from build123d import *

# Parameters (mm, degrees)
F1_DEPTH  = 38
F3_D      = 12
F5_DEPTH  = 2
F6_R      = 10
F8_D      = 10
F10_DEPTH = 2
F12_DEPTH = 2
F14_W     = 30
F14_H     = 36
F15_DEPTH = 2
F16_W     = 1
F16_H     = 15
F17_DEPTH = 5


# Not quite as in the source:
# - a feature names something its author has since deleted; it is built from what else it names


with BuildPart() as f1:
    # F0 (on Front) → F1 (new body)
    with BuildSketch(Plane.XZ):
        with BuildLine():
            Line((20, 0), (0, 0))
            Line((0, 0), (0, -2))
            Line((0, -2), (20.5, -2))
            ThreePointArc((20.5, -2), (28.6317279836, 1.3682720164), (32, 9.5))
            Line((32, 9.5), (32, 90))
            Line((32, 90), (30, 90))
            Line((30, 90), (30, 10))
            ThreePointArc((30, 10), (27.0710678119, 2.9289321881), (20, 0))
        make_face()
    extrude(amount=F1_DEPTH)

    # F3 (through all)
    with Locations(Plane.XY):
        with Locations((5, -19)):
            Hole(F3_D / 2)

    # F4 (on face) → F5 (join)
    with BuildSketch(Plane(origin=(0, 0, -2), x_dir=(1, 0, 0), z_dir=(0, 0, -1))):
        with BuildLine():
            ThreePointArc((1, 29.246950766), (6.1242290384, 29.9423996029), (11, 28.2195444573))
            ThreePointArc((11, 28.2195444573), (11.8405728739, 27.8759539642), (12.6811457479, 28.2195444573))
            ThreePointArc((12.6811457479, 28.2195444573), (7.117566826, 30.811685347), (1, 30.313708499))
            ThreePointArc((1, 30.313708499), (0.5841901068, 29.7803296325), (1, 29.246950766))
        make_face()
        with BuildLine():
            ThreePointArc((11, 9.7804555427), (6.1242290384, 8.0576003971), (1, 8.753049234))
            ThreePointArc((1, 8.753049234), (0.5841901068, 8.2196703675), (1, 7.686291501))
            ThreePointArc((1, 7.686291501), (7.117566826, 7.188314653), (12.6811457479, 9.7804555427))
            ThreePointArc((12.6811457479, 9.7804555427), (11.8405728739, 10.1240460358), (11, 9.7804555427))
        make_face()
    extrude(amount=F5_DEPTH)

    # F6
    f6_edges = [f1.edges().sort_by_distance(p)[0] for p in [
        (31, -38, 90),
        (31, 0, 90),
    ]]
    fillet(f6_edges, radius=F6_R)

    # F8 (through all)
    with Locations(Plane.YZ.offset(32)):
        with Locations((-19, 75)):
            Hole(F8_D / 2)


with BuildPart() as f10:
    # F9 (on face) → F10 (new body)
    with BuildSketch(Plane.XZ.offset(38)):
        with BuildLine():
            Line((0, 40), (0, 0))
            Line((0, 0), (20, 0))
            ThreePointArc((20, 0), (27.0710678119, 2.9289321881), (30, 10))
            Line((30, 10), (30, 40))
            Line((30, 40), (0, 40))
        make_face()
    extrude(amount=-F10_DEPTH)


with BuildPart() as f12:
    # F11 (on face) → F12 (new body)
    with BuildSketch(Plane(origin=(0, 0, 0), x_dir=(-1, 0, 0), z_dir=(0, 1, 0))):
        with BuildLine():
            Line((-20, 0), (0, 0))
            Line((0, 0), (0, 40))
            Line((0, 40), (-30, 40))
            Line((-30, 40), (-30, 10))
            ThreePointArc((-30, 10), (-27.0710678119, 2.9289321881), (-20, 0))
        make_face()
    extrude(amount=-F12_DEPTH)


with BuildPart() as f1_1:
    add(f1.part)

    # F13: union F10, F12
    add(f10.part)
    add(f12.part)

    # F14 (on face) → F15 (join)
    with BuildSketch(Plane.XY.offset(40)):
        with Locations((15, -20)):
            Rectangle(F14_W, F14_H)
    extrude(amount=-F15_DEPTH)

    # F16 (on face) → F17 (join)
    with BuildSketch(Plane(origin=(0, 0, 0), x_dir=(0, -1, 0), z_dir=(-1, 0, 0))):
        with Locations((37, 7.5)):
            Rectangle(F16_W, F16_H)
    extrude(amount=F17_DEPTH)


solid = f1_1.part
Read the model definition and answer for the solid it produces. Units are mm, in the model's axes. A direction names the side the tool comes from. Coordinates: 2 decimals unless noted, no trailing zeros. Loops run counter-clockwise (first coordinate to the right, second up) from the corner with the lowest first, then second, coordinate; pieces in that order, holes last. Notation, with made-up numbers: (-38, 81) -> (4, 81) arc R36 ccw to (4, 120) -> close; hole circle Ø1 at (-2.5, 14.25). An arc over 180 degrees is marked (long way). Write item = value, one per line. Start each with the question number.
1) The part is cut by section D-D, the plane y = -4. Determine the outline of the cut face in (x, z), plus the area to 3 significant figures.
2) The part is cut by section C-C, the plane x = 17. Determine the outline of the cut face in (y, z), plus the area to 3 significant figures.
3) Find the intervals of material crossed by L1, parallel to Z at x = 2, y = -4; L2, parallel to Y at x = 26, z = 5.5; L3, parallel to X at y = -27, z = 39.5, in increasing order. Write a range as from..to.
4) The part is cut by section B-B, the plane y = -19. Determine the outline of the cut face in (x, z), plus the area to 3 significant figures.
5) For faces 5 (the face through (11.828, -27.876, -2.986)), 6 (the face through (15, -19, 40)), 7 (the face through (7.032, -7.173, -2.986)), 8 (the face through (-2, -36.5, 7)), 9 (the face through (7.203, -30.796, -2.986)), determine the directions among +Z, -Z, +X, -X, +Y, -Y from which every point of the face is accessible in a straight line to the end or side of a thin tool.
6) Given P1, Ø4, axis at y = -31.5, z = 50, coming from the -X side; P2, Ø1, axis at x = 10, y = -27, coming from the -Z side; P3, Ø5.5, axis at x = -3, z = 7.5, coming from the +Y side, each flat-ended and moving along its own axis, determine where each tip first touches the part or whether it passes through.
7) The part is cut by section A-A, the plane z = 75. Determine the outline of the cut face in (x, y), plus the area to 3 significant figures.
8) The mould has two halves that part along X. Classify faces 1 (the face through (-2, -37.5, 7)), 2 (the face through (11.854, -10.124, -2.986)), 3 (the face through (6.197, -8.065, -2.986)), 4 (the face through (30, -19, 65)): pulls with the +X half, pulls with the -X half, needs draft (parallel to the pull), parting line crosses it, or undercut.
Result:
q1.outline = (0, -2) -> (20.5, -2) arc R11.5 ccw to (32, 9.5) -> (32, 88) -> (30, 88) -> (30, 40) -> (0, 40) -> (0, 38) -> (30, 38) -> (30, 10) arc R10 cw to (20, 0) -> (0, 0) -> close
q1.area = 293 mm²
q2.outline = (-38, -2) -> (0, -2) -> (0, 40) -> (-38, 40) -> close; hole (-36, 0) -> (-2, 0) -> (-2, 38) -> (-36, 38) -> close
q2.area = 304 mm²
q3.L1 = -2..0, 38..40
q3.L2 = -38..-36, -2..0
q3.L3 = 0..32
q4.outline = (0, 38) -> (30, 38) -> (30, 10) arc R10 cw to (20, 0) -> (11, 0) -> (11, -2) -> (20.5, -2) arc R11.5 ccw to (32, 9.5) -> (32, 70) -> (30, 70) -> (30, 40) -> (0, 40) -> close; (30, 80) -> (32, 80) -> (32, 90) -> (30, 90) -> close
q4.area = 255 mm²
q5.face_5 = -Z
q5.face_6 = +Z, -X, +Y, -Y
q5.face_7 = -Z, +Y
q5.face_8 = +Z, -Z, -X, +Y
q5.face_9 = -Z, -Y
q6.P1 = 30
q6.P2 = -2
q6.P3 = -36.5
q7.outline = (30, -38) -> (32, -38) -> (32, -24) -> (30, -24) -> close; (30, -14) -> (32, -14) -> (32, 0) -> (30, 0) -> close
q7.area = 56.0 mm²
q8.face_1 = needs draft
q8.face_2 = parting line crosses it
q8.face_3 = undercut
q8.face_4 = pulls with the -X half
